Part print with two shaded views. Sizes in mm from the minimum x, y, z corner. Coordinates: 2 decimals unless noted, no trailing zeros. Write each loop counter-clockwise with the first axis right and the second up, starting at its lowest first coordinate (ties: lowest second). Pieces come first, ordered by that corner, then holes. Notation, with made-up numbers: (74, -16.5) - (126, -16.5) arc R10 ccw to (126, -4.5) - close; hole circle Ø11 at (84.5, 13). An arc over 180 degrees is marked (long way). Answer in a Markdown table with one row per item. Add a question column.
Q1. Drill centre lines: line 1 along X through (y, z) = (11, 0.2); line 2 along Y through (x, z) = (79, 2.5); line 3 along Y through (x, z) = (70, 0.95). Where is each one in solid material? Low to high. Write a range as from..to.
Q2. Pin check, flat tip, straight feed: pin 1 (3 mm diameter, centred on x = 79, y = 5.5, fed in from -Z). Stop position of the tip, or through.
Q3. Band-saw the part on C-C (z = 1.55). State how many separate pieces and enclosed holes the cut face has, and give its area (3 significant figures).
Q4. Band-saw the part on A-A (x = 6). List the corners of the cut face in (y, z).
Q5. Band-saw the part on B-B (y = 54.5). List the corners of the cut face in (x, z), and give its area (3 significant figures).
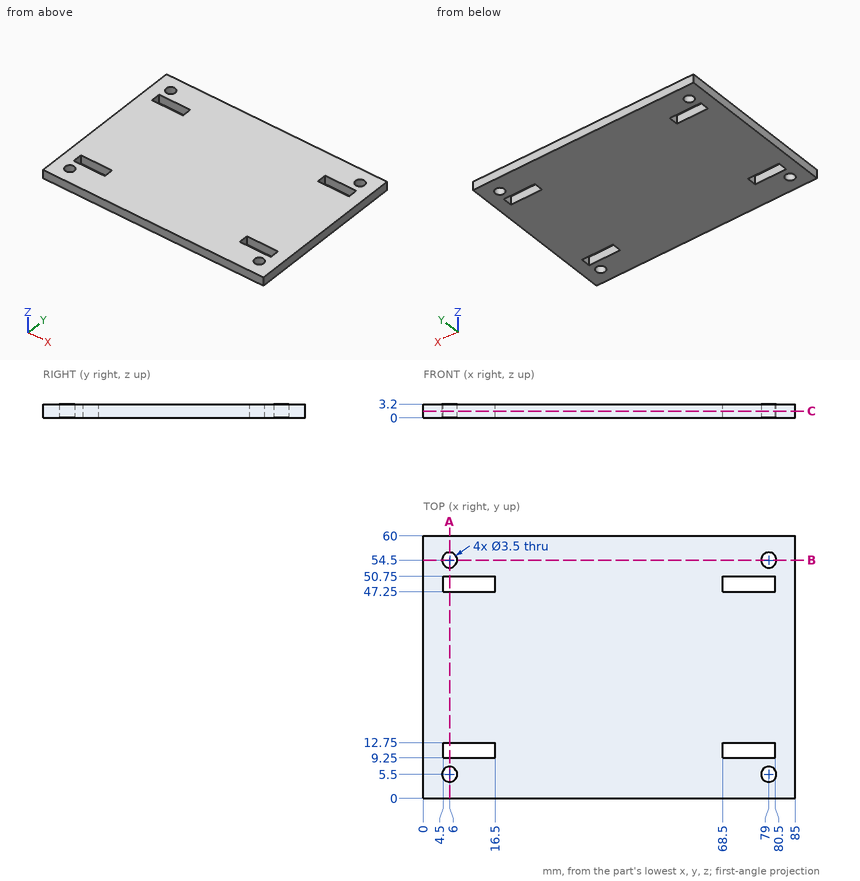
Checked values:
| question | item | result |
|---|---|---|
| 1 | line 1 | x = 0..4.5, 16.5..68.5, 80.5..85 |
| 1 | line 2 | y = 0..3.75, 7.25..9.25, 12.75..47.25, 50.75..52.75, 56.25..60 |
| 1 | line 3 | y = 0..9.25, 12.75..47.25, 50.75..60 |
| 2 | pin 1 | passes through |
| 3 | separate pieces | 1 |
| 3 | enclosed holes | 8 |
| 3 | area | 4,890 mm² |
| 4 | outline | (0, 0) - (3.75, 0) - (3.75, 3.2) - (0, 3.2) - close; (7.25, 0) - (9.25, 0) - (9.25, 3.2) - (7.25, 3.2) - close; (12.75, 0) - (47.25, 0) - (47.25, 3.2) - (12.75, 3.2) - close; (50.75, 0) - (52.75, 0) - (52.75, 3.2) - (50.75, 3.2) - close; (56.25, 0) - (60, 0) - (60, 3.2) - (56.25, 3.2) - close |
| 5 | outline | (0, 0) - (4.25, 0) - (4.25, 3.2) - (0, 3.2) - close; (7.75, 0) - (77.25, 0) - (77.25, 3.2) - (7.75, 3.2) - close; (80.75, 0) - (85, 0) - (85, 3.2) - (80.75, 3.2) - close |
| 5 | area | 250 mm² |
